Design review of the part built by this model. Coordinates are the model's own, in mm. Face numbers are marked on the shaded views. Coordinates: 2 decimals unless noted, no trailing zeros. Loops run counter-clockwise (first coordinate to the right, second up) from the corner with the lowest first, then second, coordinate; pieces in that order, holes last. Notation, with made-up numbers: (21, 88) -> (73, 88) arc R33 ccw to (73, 121) -> close; hole circle Ø11 at (43.5, 64). An arc over 180 degrees is marked (long way). Use one line per item in the form item = value. Start each with the question number.
1. Consider section B-B (x = 0). State the section outline as (y, z) points, then the cut area to 3 significant figures.
2. Consider section C-C (y = 6.75). State the section outline as (x, z) points.
3. The part is to be moulded in two halves that separate along X. For the marked faces 1 and 2, say which applies: released by +X, released by -X, zero draft, split by the parting line, or undercut.
4. Wall thickness on line 1 (X direction, y = 8.5, z = -5.5); line 2 (Z direction, x = 4, y = 8.75); line 3 (X direction, y = 5.5, z = -22.5): over which ranges is each line inside the solid? List them lowest first. Write a range as from..to.
5. For pin 1 (2 mm diameter, centred on y = 3.5, z = -6, fed in from +X); pin 2 (4 mm diameter, centred on y = 7.5, z = 28, fed in from +X); pin 3 (4 mm diameter, centred on x = -19, y = 7, fed in from +Z), all flat-tipped, find the tip position at first contact; note any pin that passes through.
6. Consider section A-A (z = 0). State how many separate pieces and enclosed holes the cut face has, then the cut area to 3 significant figures.
from build123d import *

# Parameters (mm, degrees)
CHAMFER_SIZE       = 0.5
CHAMFER001_SIZE    = 0.5
CHAMFER002_SIZE    = 0.5
CHAMFER003_SIZE    = 0.5
POCKET_DEPTH       = 275.303804
POLARPATTERN_COUNT = 3
CHAMFER004_SIZE    = 1
FILLET_R           = 1


with BuildPart() as part:
    # Sketch → Revolution (revolve)
    with BuildSketch(Plane.XY):
        with BuildLine():
            Line((-15, 9), (-47.5, 9))
            Line((-47.5, 9), (-47.5, 3))
            Line((-47.5, 3), (-22, 3))
            ThreePointArc((-19, 0), (-19.87868, 2.12132), (-22, 3))
            Line((-19, 0), (-15, 0))
            Line((-15, 0), (-15, 9))
        make_face()
    revolve(axis=Axis((0, 0, 0), (0, 1, 0)))

    # Chamfer
    chamfer_edges = [part.edges().sort_by_distance(p)[0] for p in [
        (47.5, 3, 0),
    ]]
    chamfer(chamfer_edges, length=CHAMFER_SIZE)

    # Chamfer001
    chamfer001_edges = [part.edges().sort_by_distance(p)[0] for p in [
        (47.5, 9, 0),
    ]]
    chamfer(chamfer001_edges, length=CHAMFER001_SIZE)

    # Chamfer002
    chamfer002_edges = [part.edges().sort_by_distance(p)[0] for p in [
        (15, 0, 0),
    ]]
    chamfer(chamfer002_edges, length=CHAMFER002_SIZE)

    # Chamfer003
    chamfer003_edges = [part.edges().sort_by_distance(p)[0] for p in [
        (15, 9, 0),
    ]]
    chamfer(chamfer003_edges, length=CHAMFER003_SIZE)

    # Sketch001 (on Face9 of Chamfer003) → Pocket (cut, through all)
    with BuildSketch(Plane.XZ.offset(-3)):
        with BuildLine():
            ThreePointArc((28.182522, 29.086001), (0, 40.5), (-28.182522, 29.086001))
            ThreePointArc((-28.182522, 29.086001), (-30.311454, 24.073232), (-28.203222, 19.051721))
            ThreePointArc((-28.203222, 19.051721), (-21.198816, 16.944507), (-14.272296, 19.295118))
            ThreePointArc((14.272296, 19.295118), (0, 24), (-14.272296, 19.295118))
            ThreePointArc((14.272296, 19.295118), (21.198816, 16.944507), (28.203222, 19.051721))
            ThreePointArc((28.203222, 19.051721), (30.311454, 24.073232), (28.182522, 29.086001))
        make_face()
    pocket = extrude(amount=-POCKET_DEPTH, mode=Mode.SUBTRACT)

    # PolarPattern: Pocket ×3 about axis
    polarpattern_axis = Axis((0, 3, 0), (0, -1, 0))
    for i in range(1, POLARPATTERN_COUNT):
        add(pocket.rotate(polarpattern_axis, i * 360 / POLARPATTERN_COUNT), mode=Mode.SUBTRACT)

    # Chamfer004
    chamfer004_edges = [part.edges().sort_by_distance(p)[0] for p in [
        (-35.074029, 3, -20.25),
    ]]
    chamfer(chamfer004_edges, length=CHAMFER004_SIZE)

    # Fillet
    fillet_edges = [part.edges().sort_by_distance(p)[0] for p in [
        (0, 3, 40.5),
    ]]
    fillet(fillet_edges, radius=FILLET_R)


solid = part.part
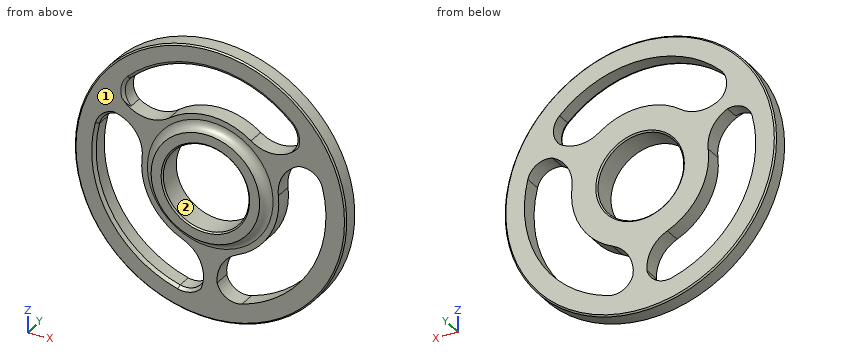
Geometry check:
q1.outline = (0, -19) arc R3 cw to (3, -22) -> (3, -47) -> (3.5, -47.5) -> (8.5, -47.5) -> (9, -47) -> (9, -15.5) -> (8.5, -15) -> (0.5, -15) -> (0, -15.5) -> close; (0, 15.5) -> (0.5, 15) -> (8.5, 15) -> (9, 15.5) -> (9, 24) -> (3, 24) -> (3, 22) arc R3 cw to (0, 19) -> close; (3, 41.5) arc R1 ccw to (4, 40.5) -> (9, 40.5) -> (9, 47) -> (8.5, 47.5) -> (3.5, 47.5) -> (3, 47) -> close
q1.area = 318 mm²
q2.outline = circle Ø95 at (0, 0); hole (-39.28, 9.86) arc R40.5 ccw to (-11.1, -38.95) arc R7 ccw to (-2.4, -33.95) arc R12 ccw to (-9.57, -22.01) arc R24 cw to (-23.85, 2.71) arc R12 ccw to (-30.6, 14.9) arc R7 ccw to start; hole (-28.2, 19.05) arc R12 ccw to (-14.27, 19.3) arc R24 cw to (14.27, 19.3) arc R12 ccw to (28.2, 19.05) arc R7 ccw to (28.18, 29.09) arc R40.5 ccw to (-28.18, 29.09) arc R7 ccw to start; hole circle Ø30 at (0, 0); hole (2.4, -33.95) arc R7 ccw to (11.1, -38.95) arc R40.5 ccw to (39.28, 9.86) arc R7 ccw to (30.6, 14.9) arc R12 ccw to (23.85, 2.71) arc R24 cw to (9.57, -22.01) arc R12 ccw to start
q3.face_1 = zero draft
q3.face_2 = undercut
q4.line_1 = -47.18..-40.12, -23.36..-13.96, 13.96..23.36, 40.12..47.18
q4.line_2 = -47.08..-36.93, -26.96..-14.72, 14.72..23.66, 40.3..47.08
q4.line_3 = -41.83..-33.67, -8.57..8.57, 33.67..41.83
q5.pin_1 = 47.24
q5.pin_2 = 39.75
q5.pin_3 = 44.35
q6.separate_pieces = 4
q6.enclosed_holes = 0
q6.area = 218 mm²
